For this review, use the dimensioned drawing (mm, ordinates from the lowest corner) and the shaded views. Coordinates: 2 decimals unless noted, no trailing zeros. Order: outer loops, then holes, each group sorted by start corner. A loop starts at its lowest first (then second) coordinate and runs counter-clockwise, first axis right, second up. Notation, with made-up numbers: (15, 21) -> (27, 21) arc R27 ccw to (27, 56) -> close; hole circle Ø2 at (53.5, 2.25). An arc over 180 degrees is marked (long way). Use one line per item in the form item = value. Start each with the question number.
(1) Take a section at B-B (x = 4). State the section outline as (y, z) points (1 decimal).
(2) Insertion check: pin 1 Ø3 at (x, z) = (36.53, 36.53) entering from +Y; pin 2 Ø1 at (x, y) = (26, 2.5) entering from +Z (1 decimal). Each pin has a flat end and moves straight along its axis. Give the tip position at first contact, or say it passes through.
(3) Take a section at A-A (z = 4). State the section outline as (x, y) points (1 decimal).
(4) Take a section at D-D (z = 30.5). State the section outline as (x, y) points.
(5) Take a section at C-C (y = 2.3). State the section outline as (x, z) points (1 decimal).
(6) Wall thickness on line 1 along X through (y, z) = (1.65, 4) (1 decimal); line 2 along Z through (x, y) = (37, 2.6) (1 decimal); line 3 along Z through (x, y) = (14, 0.6) (1 decimal): over which ranges is each line inside the solid? List them lowest first.
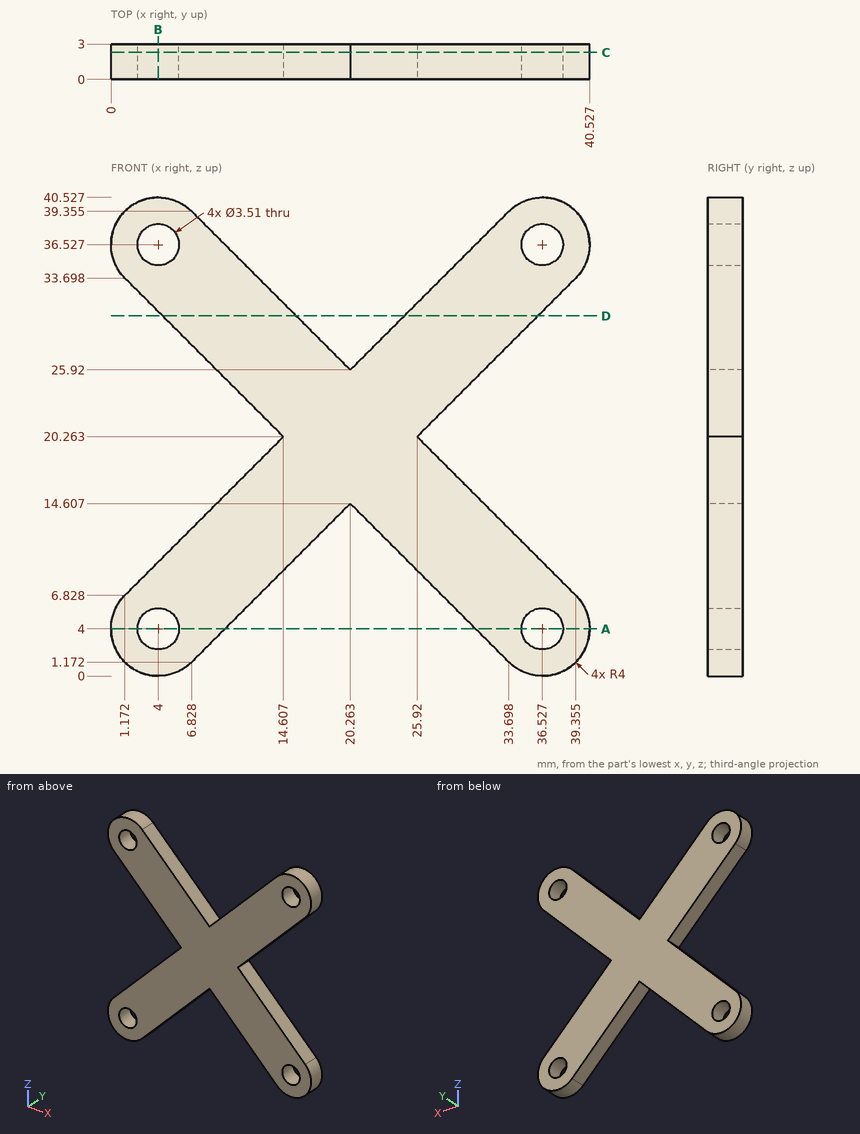
Findings:
q1.outline = (0, 0) -> (3, 0) -> (3, 2.2) -> (0, 2.2) -> close; (0, 5.8) -> (3, 5.8) -> (3, 9.7) -> (0, 9.7) -> close; (0, 30.9) -> (3, 30.9) -> (3, 34.8) -> (0, 34.8) -> close; (0, 38.3) -> (3, 38.3) -> (3, 40.5) -> (0, 40.5) -> close
q2.pin_1 = through
q2.pin_2 = 32.2
q3.outline = (0, 0) -> (2.2, 0) -> (2.2, 3) -> (0, 3) -> close; (5.8, 0) -> (9.7, 0) -> (9.7, 3) -> (5.8, 3) -> close; (30.9, 0) -> (34.8, 0) -> (34.8, 3) -> (30.9, 3) -> close; (38.3, 0) -> (40.5, 0) -> (40.5, 3) -> (38.3, 3) -> close
q4.outline = (4.37, 0) -> (15.68, 0) -> (15.68, 3) -> (4.37, 3) -> close; (24.84, 0) -> (36.16, 0) -> (36.16, 3) -> (24.84, 3) -> close
q5.outline = (1.2, 6.8) arc R4 ccw to (6.8, 1.2) -> (20.3, 14.6) -> (33.7, 1.2) arc R4 ccw to (39.4, 6.8) -> (25.9, 20.3) -> (39.4, 33.7) arc R4 ccw to (33.7, 39.4) -> (20.3, 25.9) -> (6.8, 39.4) arc R4 ccw to (1.2, 33.7) -> (14.6, 20.3) -> close; hole circle Ø3.5 at (4, 4); hole circle Ø3.5 at (4, 36.5); hole circle Ø3.5 at (36.5, 4); hole circle Ø3.5 at (36.5, 36.5)
q6.line_1 = 0 to 2.2, 5.8 to 9.7, 30.9 to 34.8, 38.3 to 40.5
q6.line_2 = 0 to 2.3, 5.7 to 9.2, 31.3 to 34.8, 38.2 to 40.5
q6.line_3 = 8.3 to 19.7, 20.9 to 32.2
